Read the model definition and answer for the solid it produces. Units are mm, in the model's axes. A direction names the side the tool comes from. Coordinates: 2 decimals unless noted, no trailing zeros. Write each loop counter-clockwise with the first axis right and the second up, starting at its lowest first coordinate (ties: lowest second). Pieces come first, ordered by that corner, then holes. Notation, with made-up numbers: (-10.5, 63) - (28.5, 63) arc R19 cw to (28.5, 87) - close; hole circle Ø9 at (-31, -37.5). An arc over 180 degrees is marked (long way). Return JSON: item names as keys, results as strings.
```python
from build123d import *

# Parameters (mm, degrees)
F0_R     = 1.5
F1_DEPTH = 4
F2_R     = 2
F3_R     = 1
F4_R     = 3
F5_W     = 12.076094228
F5_H     = 2
F6_DEPTH = 2
F7_R     = 1


with BuildPart() as f1:
    # F0 (on Top) → F1 (new body)
    with BuildSketch(Plane.XY):
        Polygon((0, 19.8), (-2.75, 16.6034741081), (-2.75, -1.4034741081), (0, -4.6), (21.5, -4.6), (24.25, -1.4034741081), (24.25, 16.6034741081), (21.5, 19.8), align=None)
        Circle(F0_R, mode=Mode.SUBTRACT)
        with Locations((21.5, 0)):
            Circle(F0_R, mode=Mode.SUBTRACT)
        with Locations((0, 15.2)):
            Circle(F0_R, mode=Mode.SUBTRACT)
        with BuildLine():
            Line((20.6041763566, -2.6), (0.8958236434, -2.6))
            ThreePointArc((0.8958236434, -2.6), (2.712240771, 0.4541475531), (0, 2.75))
            Line((0, 2.75), (0, 12.45))
            ThreePointArc((0, 12.45), (2.712240771, 14.7458524469), (0.8958236434, 17.8))
            Line((0.8958236434, 17.8), (20.6041763566, 17.8))
            ThreePointArc((20.6041763566, 17.8), (18.787759229, 14.7458524469), (21.5, 12.45))
            Line((21.5, 12.45), (21.5, 2.75))
            ThreePointArc((21.5, 2.75), (18.787759229, 0.4541475531), (20.6041763566, -2.6))
        make_face(mode=Mode.SUBTRACT)
        with Locations((21.5, 15.2)):
            Circle(F0_R, mode=Mode.SUBTRACT)
    extrude(amount=F1_DEPTH)

    # F2
    f2_edges = [f1.edges().sort_by_distance(p)[0] for p in [
        (0.895824, 17.8, 2),
        (20.604176, 17.8, 2),
        (0.895824, -2.6, 2),
        (20.604176, -2.6, 2),
    ]]
    fillet(f2_edges, radius=F2_R)

    # F3
    f3_edges = [f1.edges().sort_by_distance(p)[0] for p in [
        (0, 12.45, 2),
        (0, 2.75, 2),
        (21.5, 12.45, 2),
        (21.5, 2.75, 2),
    ]]
    fillet(f3_edges, radius=F3_R)

    # F4
    f4_edges = [f1.edges().sort_by_distance(p)[0] for p in [
        (0, -4.6, 2),
        (21.5, -4.6, 2),
        (24.25, -1.403474, 2),
        (24.25, 16.603474, 2),
        (21.5, 19.8, 2),
        (0, 19.8, 2),
        (-2.75, 16.603474, 2),
        (-2.75, -1.403474, 2),
    ]]
    fillet(f4_edges, radius=F4_R)

    # F5 (on face) → F6 (cut)
    with BuildSketch(Plane(origin=(0, 0, 0), x_dir=(1, 0, 0), z_dir=(0, 0, -1))):
        with Locations((10.75, -18.8)):
            Rectangle(F5_W, F5_H)
        with BuildLine():
            Line((3.211952886, 4.6), (3.211952886, 1.9228756555))
            ThreePointArc((3.211952886, 1.9228756555), (3.8890772305, 2.4228756555), (4.711952886, 2.6))
            Line((4.711952886, 2.6), (16.788047114, 2.6))
            ThreePointArc((16.788047114, 2.6), (17.6109227695, 2.4228756555), (18.288047114, 1.9228756555))
            Line((18.288047114, 1.9228756555), (18.288047114, 4.6))
            Line((18.288047114, 4.6), (3.211952886, 4.6))
        make_face()
    extrude(amount=-F6_DEPTH, mode=Mode.SUBTRACT)

    # F7
    f7_edges = [f1.edges().sort_by_distance(p)[0] for p in [
        (4.711953, 18.8, 2),
        (16.788047, 18.8, 2),
        (18.288047, -3.261438, 2),
        (3.211953, -3.261438, 2),
    ]]
    fillet(f7_edges, radius=F7_R)


solid = f1.part
```
(1) A cutting plane is placed at C-C (y = -1). Determine the outline of the cut face in (x, z), and give its area (3 significant figures).
Answer:
{"outline": "(-2.66, 0) - (-1.12, 0) - (-1.12, 4) - (-2.66, 4) - close; (1.12, 0) - (2.75, 0) - (2.75, 4) - (1.12, 4) - close; (18.75, 0) - (20.38, 0) - (20.38, 4) - (18.75, 4) - close; (22.62, 0) - (24.16, 0) - (24.16, 4) - (22.62, 4) - close", "area": "25.4 mm²"}
(2) Flat-ended cylindrical pins translate along their axes: P1, Ø0.6, axis at x = 8.5, y = -3.5, coming from the -Z side; P2, Ø2.5, axis at x = 21.5, y = 15.2, coming from the -Z side; P3, Ø0.8, axis at y = -3.5, z = 0.5, coming from the +X side; P4, Ø1.1, axis at y = 18.5, z = 0.5, coming from the -X side. Find the tip coordinate at first contact, or state that the pin passes through.
Answer:
{"P1": "z = 2", "P2": "through", "P3": "x = 22.79", "P4": "x = -1.59"}
(3) A cutting plane is placed at D-D (z = 1.6). State how many separate pieces and enclosed holes the cut face has, and give its area (3 significant figures).
Answer:
{"separate pieces": "2", "enclosed holes": "4", "area": "176 mm²"}
(4) Determine the mould class of faces 1 (the face through (0.11, 19.52, 2.03)), 2 (the face through (21.5, 8, 2)), 3 (the face through (19.195, 13.7, 1.972)), 4 (the face through (22, 8, 0)) for opening direction X: +X half, -X half, draft (parallel to the pull), parting line (faces both ways), or undercut.
Answer:
{"face 1": "-X half", "face 2": "undercut", "face 3": "undercut", "face 4": "draft"}
(5) Which of the six approach directions +Z, -Z, +X, -X, +Y, -Y give full straight-line access (tool end or side, diameter ignored) to faces 5 (the face through (16.788, 18.8, 0.5)), 6 (the face through (18, -3.3, 1.7)), 7 (the face through (24.068, -1.32, 2.028)), 8 (the face through (11, -4.6, 3)), 9 (the face through (18.305, 17.104, 2.028))?
Answer:
{"face 5": "-Z, +Y, -Y", "face 6": "-Z, -Y", "face 7": "+Z, -Z, +X, -Y", "face 8": "+Z, -Z, +X, -X, -Y", "face 9": "+Z, -Z"}
(6) Straight lines are drawn through the part: line 1 (X direction, y = 11, z = 2.95); line 2 (Y direction, x = 5.25, z = 3.3); line 3 (X direction, y = 15.25, z = 1.35). For each, find the intervals that lie inside material, in ascending order. Write a range as from..to.
Answer:
{"line 1": "-2.75..0, 21.5..24.25", "line 2": "-4.6..-2.6, 17.8..19.8", "line 3": "-2.75..-1.5, 1.5..2.75, 18.75..20, 23..24.25"}
(7) A cutting plane is placed at B-B (y = 9.5). Determine the outline of the cut face in (x, z), and give its area (3 significant figures).
Answer:
{"outline": "(-2.75, 0) - (0, 0) - (0, 4) - (-2.75, 4) - close; (21.5, 0) - (24.25, 0) - (24.25, 4) - (21.5, 4) - close", "area": "22.0 mm²"}
(8) A cutting plane is placed at A-A (x = 10.5). Determine the outline of the cut face in (y, z).
Answer:
{"outline": "(-4.6, 2) - (-2.6, 2) - (-2.6, 4) - (-4.6, 4) - close; (17.8, 2) - (19.8, 2) - (19.8, 4) - (17.8, 4) - close"}
